from build123d import *

# Parameters (mm, degrees)
SKETCH1_W            = 5.41
SKETCH1_H            = 5.41
SKETCH1_W_2          = 4.549942703
SKETCH1_H_2          = 4.549942703
SKETCH1_W_3          = 0.44
BOSS_EXTRUDE8_DEPTH  = 8.9
SKETCH2_W            = 0.25
SKETCH2_H            = 3.415060647
SKETCH2_H_2          = 1.584939353
CUT_EXTRUDE1_DEPTH   = 1
SKETCH3_W            = 2
SKETCH3_H            = 0.168194263
BOSS_EXTRUDE9_DEPTH  = 0.44
BOSS_EXTRUDE10_DEPTH = 2
SKETCH6_W            = 3.011984057
SKETCH6_H            = 5.99945952
CUT_EXTRUDE2_DEPTH   = 10


# Read off the part's stored shape, not the designer's step: Mirror10
with BuildPart() as part:
    # Sketch1 → Boss-Extrude8 (new body)
    # profile 1 of 10: a face of its own
    with BuildSketch(Plane(origin=(61.037479951, 0, 196.423934756), x_dir=(1, 0, 0), z_dir=(0, 1, 0))):
        with Locations((-39.807700339, 14.550827763)):
            Rectangle(SKETCH1_W, SKETCH1_H)
        with Locations((-39.797728988, 14.560799114)):
            Rectangle(SKETCH1_W_2, SKETCH1_H_2, mode=Mode.SUBTRACT)
    # profile 2 of 10: a face of its own
    with BuildSketch(Plane(origin=(61.037479951, 0, 196.423934756), x_dir=(1, 0, 0), z_dir=(0, 1, 0))):
        with Locations((-39.807700339, 14.560799114)):
            Rectangle(SKETCH1_W_3, SKETCH1_H_2)
    # profile 3 of 10: a face of its own
    with BuildSketch(Plane(origin=(61.037479951, 0, 196.423934756), x_dir=(1, 0, 0), z_dir=(0, 1, 0))):
        with BuildLine():
            ThreePointArc((-42.092643043, 17.255827763), (-42.302671691, 17.470827763), (-42.512700339, 17.255827763))
            Line((-42.512700339, 17.255827763), (-42.092643043, 17.255827763))
        make_face()
    # profile 4 of 10: a face of its own
    with BuildSketch(Plane(origin=(61.037479951, 0, 196.423934756), x_dir=(1, 0, 0), z_dir=(0, 1, 0))):
        with BuildLine():
            ThreePointArc((-42.512700339, 17.255827763), (-42.722700339, 17.035827763), (-42.512700339, 16.815827763))
            Line((-42.512700339, 16.815827763), (-42.512700339, 17.255827763))
        make_face()
    # profile 5 of 10: a face of its own
    with BuildSketch(Plane(origin=(61.037479951, 0, 196.423934756), x_dir=(1, 0, 0), z_dir=(0, 1, 0))):
        with BuildLine():
            ThreePointArc((-42.512700339, 12.285827763), (-42.722700339, 12.065827763), (-42.512700339, 11.845827763))
            Line((-42.512700339, 11.845827763), (-42.512700339, 12.285827763))
        make_face()
    # profile 6 of 10: a face of its own
    with BuildSketch(Plane(origin=(61.037479951, 0, 196.423934756), x_dir=(1, 0, 0), z_dir=(0, 1, 0))):
        with BuildLine():
            Line((-42.092643043, 11.845827763), (-42.512700339, 11.845827763))
            ThreePointArc((-42.512700339, 11.845827763), (-42.302671691, 11.630827763), (-42.092643043, 11.845827763))
        make_face()
    # profile 7 of 10: a face of its own
    with BuildSketch(Plane(origin=(61.037479951, 0, 196.423934756), x_dir=(1, 0, 0), z_dir=(0, 1, 0))):
        with BuildLine():
            Line((-37.102700339, 11.845827763), (-37.522757636, 11.845827763))
            ThreePointArc((-37.522757636, 11.845827763), (-37.312728988, 11.630827763), (-37.102700339, 11.845827763))
        make_face()
    # profile 8 of 10: a face of its own
    with BuildSketch(Plane(origin=(61.037479951, 0, 196.423934756), x_dir=(1, 0, 0), z_dir=(0, 1, 0))):
        with BuildLine():
            Line((-37.102700339, 12.285827763), (-37.102700339, 11.845827763))
            ThreePointArc((-37.102700339, 11.845827763), (-36.892700339, 12.065827763), (-37.102700339, 12.285827763))
        make_face()
    # profile 9 of 10: a face of its own
    with BuildSketch(Plane(origin=(61.037479951, 0, 196.423934756), x_dir=(1, 0, 0), z_dir=(0, 1, 0))):
        with BuildLine():
            ThreePointArc((-37.102700339, 17.255827763), (-37.312728988, 17.470827763), (-37.522757636, 17.255827763))
            Line((-37.522757636, 17.255827763), (-37.102700339, 17.255827763))
        make_face()
    # profile 10 of 10: a face of its own
    with BuildSketch(Plane(origin=(61.037479951, 0, 196.423934756), x_dir=(1, 0, 0), z_dir=(0, 1, 0))):
        with BuildLine():
            Line((-37.102700339, 17.255827763), (-37.102700339, 16.815827763))
            ThreePointArc((-37.102700339, 16.815827763), (-36.892700339, 17.035827763), (-37.102700339, 17.255827763))
        make_face()
    extrude(amount=BOSS_EXTRUDE8_DEPTH)

    # Sketch2 → Cut-Extrude1 (cut)
    with BuildSketch(Plane(origin=(23.934779612, 0, 196.423934756), x_dir=(0, 0, -1), z_dir=(1, 0, 0))):
        with Locations((13.425827763, 5.607530324)):
            Rectangle(SKETCH2_W, SKETCH2_H)
        with Locations((13.425827763, 8.107530324)):
            Rectangle(SKETCH2_W, SKETCH2_H_2)
        with Locations((15.675827763, 8.107530324)):
            Rectangle(SKETCH2_W, SKETCH2_H_2)
        with Locations((15.675827763, 5.607530324)):
            Rectangle(SKETCH2_W, SKETCH2_H)
    extrude(amount=-CUT_EXTRUDE1_DEPTH, mode=Mode.SUBTRACT)

    # Sketch3 → Boss-Extrude9 (add)
    with BuildSketch(Plane(origin=(23.934779612, 0, 196.423934756), x_dir=(0, 0, -1), z_dir=(1, 0, 0))):
        with Locations((14.550827763, 6.984097132)):
            Rectangle(SKETCH3_W, SKETCH3_H)
    extrude(amount=BOSS_EXTRUDE9_DEPTH)

    # Sketch5 → Boss-Extrude10 (add)
    with BuildSketch(Plane(origin=(61.037479951, 0, 182.873106993), x_dir=(1, 0, 0), z_dir=(0, 0, 1))):
        Polygon((-36.662700339, 7.068194263), (-37.102700339, 8.9), (-37.102700339, 7.068194263), align=None)
    extrude(amount=-BOSS_EXTRUDE10_DEPTH)

    # Sketch6 → Cut-Extrude2 (cut)
    with BuildSketch(Plane(origin=(61.037479951, 8.9, 196.423934756), x_dir=(1, 0, 0), z_dir=(0, 1, 0))):
        with Locations((-41.313692367, 14.541370124)):
            Rectangle(SKETCH6_W, SKETCH6_H)
    extrude(amount=-CUT_EXTRUDE2_DEPTH, mode=Mode.SUBTRACT)

    # Mirror10: part across plane


with BuildPart() as part_1:
    add(part.part)
    add(part.part.mirror(Plane(origin=(21.229779612, -1.1, 178.882834872), x_dir=(0, 0, 1), z_dir=(1, 0, 0))))


solid = part_1.part
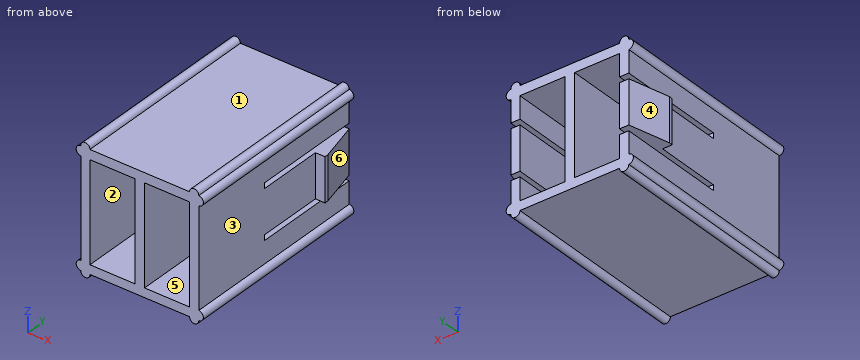
Geometry check sheet. Reference: the model listing, model coordinates, mm. Face numbers are marked on the shaded views. A direction names the side the tool comes from. Coordinates: 2 decimals unless noted, no trailing zeros. Order: outer loops, then holes, each group sorted by start corner. A loop starts at its lowest first (then second) coordinate and runs counter-clockwise, first axis right, second up. Notation, with made-up numbers: (12, 66.25) - (67, 66.25) arc R17 cw to (67, 94.25) - close; hole circle Ø10 at (-15, 37). An arc over 180 degrees is marked (long way). Answer in a Markdown table with one row per item. Add a question column.
1) Material ranges on line 1 along X through (y, z) = (3.75, 181.65); line 2 along Z through (x, y) = (21.5, 1.5); line 3 along Z through (x, y) = (21.25, 6.5), recorded low to high. Write a range as [from, to].
2) Set-up check for the marked faces 1, 2 and 3: record each of +Z, -Z, +X, -X, +Y, -Y from which the full face is reachable in a straight line by a thin tool's end or side.
3) Cross-section at B-B, the plane x = 19.5. Record the cut outline in (y, z).
4) Gauge pin test, flat ends, axial feed: P1, Ø0.6, axis at x = 22.5, y = 5.5, coming from the -Z side; P2, Ø1, axis at x = 22, y = 3, coming from the +Z side; P3, Ø3.5, axis at y = 4.5, z = 183, coming from the -X side. Record the tip position at first contact, or that the pin passes through.
5) Cross-section at C-C, the plane y = 1.5. Record the cut outline in (x, z), then the cut area to 3 significant figures.
6) Release check for a two-part mould opening along X. For the marked faces 4, 5 and 6 record: +X half, -X half, draft (parallel to the pull), parting line (faces both ways), or undercut.
7) Cross-section at A-A, the plane z = 183.8. Record the cut outline in (x, y), then the cut area to 3 significant figures.
8) Cross-section at D-D, the plane z = 181.2. Record the cut outline in (x, y), then the cut area to 3 significant figures.
Check result:
| question | item | result |
|---|---|---|
| 1 | line 1 | x = [18.52, 18.94], [21.01, 21.45], [23.51, 23.93] |
| 1 | line 2 | z = [179.17, 179.59], [184.14, 184.58] |
| 1 | line 3 | z = [179.17, 184.58] |
| 2 | face 1 | +Z, +Y, -Y |
| 2 | face 2 | +Y, -Y |
| 2 | face 3 | +X, -Y |
| 3 | outline | (0, 179.17) - (8.9, 179.17) - (8.9, 179.59) - (0, 179.59) - close; (0, 184.14) - (8.9, 184.14) - (8.9, 184.58) - (0, 184.58) - close |
| 4 | P1 | stops at z = 179.17 |
| 4 | P2 | stops at z = 184.58 |
| 4 | P3 | stops at x = 18.31 |
| 5 | outline | (18.52, 179.17) arc R0.21 ccw (long way) to (18.94, 179.17) - (23.51, 179.17) arc R0.21 ccw (long way) to (23.93, 179.17) arc R0.22 ccw to (23.93, 179.61) - (23.93, 184.14) arc R0.22 ccw to (23.93, 184.58) arc R0.21 ccw (long way) to (23.51, 184.58) - (18.94, 184.58) arc R0.21 ccw (long way) to (18.52, 184.58) arc R0.22 ccw to (18.52, 184.14) - (18.52, 179.61) arc R0.22 ccw to start; hole (18.94, 179.59) - (21.01, 179.59) - (21.01, 184.14) - (18.94, 184.14) - close; hole (21.45, 179.59) - (23.51, 179.59) - (23.51, 184.14) - (21.45, 184.14) - close |
| 5 | area | 11.0 mm² |
| 6 | face 4 | -X half |
| 6 | face 5 | undercut |
| 6 | face 6 | +X half |
| 7 | outline | (18.52, 0) - (18.94, 0) - (18.94, 8.9) - (18.52, 8.9) - close; (21.01, 0) - (21.45, 0) - (21.45, 8.9) - (21.01, 8.9) - close; (23.51, 0) - (23.93, 0) - (23.93, 8.9) - (23.51, 8.9) - close |
| 7 | area | 11.4 mm² |
| 8 | outline | (18.08, 6.9) - (18.52, 6.9) - (18.52, 0) - (18.94, 0) - (18.94, 8.9) - (18.52, 8.9) - (18.08, 7.07) - close; (21.01, 0) - (21.45, 0) - (21.45, 8.9) - (21.01, 8.9) - close; (23.51, 0) - (23.93, 0) - (23.93, 6.9) - (24.37, 6.9) - (24.37, 7.07) - (23.93, 8.9) - (23.51, 8.9) - close |
| 8 | area | 12.3 mm² |
